from build123d import *

# Parameters (mm, degrees)
ESTRUSIONE_ESTRUSIONE1_DEPTH = 90
FORO_6_5_6_5_1_D             = 6.5
FORO_6_5_6_5_2_D             = 6.5
FORO_6_5_6_5_2_DEPTH         = 5
FORO_6_5_6_5_2_TIP           = 1.952797012


with BuildPart() as part:
    # Schizzo1 → Estrusione-Estrusione1 (new body)
    with BuildSketch(Plane.XY):
        Polygon((0, 0), (0, 50), (5, 50), (5, 5), (50, 5), (50, 0), align=None)
    extrude(amount=ESTRUSIONE_ESTRUSIONE1_DEPTH)

    # Foro Ø6.5 (6.5)-1 (through all)
    with Locations(Plane(origin=(0, 0, 0), x_dir=(-1, 0, 0), z_dir=(0, -1, 0))):
        with Locations((-17, -82), (-42, -82)):
            Hole(FORO_6_5_6_5_1_D / 2)

    # Foro Ø6.5 (6.5)-2
    with Locations(Plane.ZY):
        with Locations((82, 42), (82, 17)):
            Hole(FORO_6_5_6_5_2_D / 2, depth=FORO_6_5_6_5_2_DEPTH)
            with Locations((0, 0, -(FORO_6_5_6_5_2_DEPTH + FORO_6_5_6_5_2_TIP / 2))):  # 118° drill point
                Cone(0, FORO_6_5_6_5_2_D / 2, FORO_6_5_6_5_2_TIP, mode=Mode.SUBTRACT)


solid = part.part
Design review of the part built by this model. Coordinates are the model's own, in mm. A direction names the side the tool comes from. Coordinates: 2 decimals unless noted, no trailing zeros. Order: outer loops, then holes, each group sorted by start corner. A loop starts at its lowest first (then second) coordinate and runs counter-clockwise, first axis right, second up.
Item 1: Take a section at A-A, the plane x = 42. Write out the cut boundary in (y, z), then the cut area to 4 significant figures.
Item 2: For pin 1 Ø10.5 at (x, z) = (17, 82) entering from +Y; pin 2 Ø4 at (y, z) = (8, 13) entering from +X, all flat-tipped, find the tip position at first contact; note any pin that passes through.
Item 3: Take a section at C-C, the plane z = 82. Write out the cut boundary in (x, y), then the cut area to 3 significant figures.
Item 4: The part is to be moulded in two halves that separate along X. For faces 1 (the cylindrical face through (16.295, 2.535, 85.173)), 2 (the flat face through (0, 25, 44)), 3 (the flat face through (14, 4.7, 0)), 4 (the cylindrical face through (43.5, 2.535, 84.883)), say which applies: pulls with the +X half, pulls with the -X half, needs draft (parallel to the pull), parting line crosses it, or undercut.
Item 5: Take a section at D-D, the plane z = 28. Write out the cut boundary in (x, y), then the cut area to 3 significant figures.
Item 6: For faces 5 (the flat face through (5, 28, 44)), 6 (the flat face through (2, 50, 44)), list the 3-axis set-ups (+Z, -Z, +X, -X, +Y, -Y) from which the entire face can be reached by the end or side of a thin tool; tool diameter is ignored.
Item 7: For line 1 (Y direction, x = 3.45, z = 82); line 2 (Z direction, x = 42, y = 2); line 3 (Y direction, x = 25, z = 24.5), list the stretches that pass through material, from the lowest coordinate up.
The answers:
1. outline: (0, 0) - (5, 0) - (5, 78.75) - (0, 78.75) - close; (0, 85.25) - (5, 85.25) - (5, 90) - (0, 90) - close
1. area: 417.5 mm2
2. pin 1: stops at y = 5
2. pin 2: stops at x = 5
3. outline: (0, 0) - (13.75, 0) - (13.75, 5) - (5, 5) - (5, 13.75) - (0, 13.75) - close; (0, 20.25) - (5, 20.25) - (5, 38.75) - (0, 38.75) - close; (0, 45.25) - (5, 45.25) - (5, 50) - (0, 50) - close; (20.25, 0) - (38.75, 0) - (38.75, 5) - (20.25, 5) - close; (45.25, 0) - (50, 0) - (50, 5) - (45.25, 5) - close
3. area: 345 mm2
4. face 1: undercut
4. face 2: pulls with the -X half
4. face 3: needs draft
4. face 4: undercut
5. outline: (0, 0) - (50, 0) - (50, 5) - (5, 5) - (5, 50) - (0, 50) - close
5. area: 475 mm2
6. face 5: +Z, -Z, +X, +Y
6. face 6: +Z, -Z, +X, -X, +Y
7. line 1: y = 0 to 13.75, 20.25 to 38.75, 45.25 to 50
7. line 2: z = 0 to 78.75, 85.25 to 90
7. line 3: y = 0 to 5
